from build123d import *

# Parameters (mm, degrees)
BOSS_EXTRUDE1_DEPTH = 20
BOSS_EXTRUDE2_START = 10
BOSS_EXTRUDE2_DEPTH = 10
SKETCH4_R           = 2.6
CUT_EXTRUDE2_DEPTH  = 6
CUT_EXTRUDE3_REACH  = 49.399
SKETCH2_R           = 6.6


with BuildPart() as part:
    # Sketch1 → Boss-Extrude1 (new body)
    with BuildSketch(Plane.XY):
        with BuildLine():
            Line((-33.49686368, 14.646798017), (16.10313632, 14.646798017))
            ThreePointArc((16.10313632, 14.646798017), (16.951664458, 14.295326155), (17.30313632, 13.446798017))
            Line((17.30313632, 13.446798017), (17.30313632, -25.353201983))
            Line((17.30313632, -25.353201983), (-34.69686368, -25.353201983))
            Line((-34.69686368, -25.353201983), (-34.69686368, 13.446798017))
            ThreePointArc((-34.69686368, 13.446798017), (-34.345391817, 14.295326155), (-33.49686368, 14.646798017))
        make_face()
    extrude(amount=-BOSS_EXTRUDE1_DEPTH)

    # Sketch3 → Boss-Extrude2 (add)
    with BuildSketch(Plane.XY.offset(BOSS_EXTRUDE2_START)):
        with BuildLine():
            Line((17.30313632, -25.353201983), (17.30313632, 13.446798017))
            ThreePointArc((17.30313632, 13.446798017), (16.951664458, 14.295326155), (16.10313632, 14.646798017))
            Line((16.10313632, 14.646798017), (-33.49686368, 14.646798017))
            ThreePointArc((-33.49686368, 14.646798017), (-34.345391817, 14.295326155), (-34.69686368, 13.446798017))
            Line((-34.69686368, 13.446798017), (-34.69686368, -25.353201983))
            Line((-34.69686368, -25.353201983), (17.30313632, -25.353201983))
        make_face()
    extrude(amount=-BOSS_EXTRUDE2_DEPTH)

    # Sketch4 → Cut-Extrude2 (cut)
    with BuildSketch(Plane(origin=(0, 14.646798017, 0), x_dir=(1, 0, 0), z_dir=(0, 1, 0))):
        with Locations(Location((-27.29686368, 5, 0), (0, 0, 270))):
            Circle(SKETCH4_R)
        with Locations(Location((-15.69686368, 5, 0), (0, 0, 270))):
            Circle(SKETCH4_R)
        with Locations(Location((-8.69686368, 12, 0), (0, 0, 270))):
            Circle(SKETCH4_R)
        with Locations(Location((-8.69686368, -2, 0), (0, 0, 270))):
            Circle(SKETCH4_R)
        with Locations(Location((-1.69686368, 5, 0), (0, 0, 270))):
            Circle(SKETCH4_R)
        with Locations(Location((9.90313632, 5, 0), (0, 0, 270))):
            Circle(SKETCH4_R)
    extrude(amount=-CUT_EXTRUDE2_DEPTH, mode=Mode.SUBTRACT)

    # Sketch2 → Cut-Extrude3 (cut, up to next)
    with BuildSketch(Plane.XY, mode=Mode.PRIVATE) as cut_extrude3_sk1:
        with Locations((-8.69686368, -5.353201983)):
            Circle(SKETCH2_R)
    cut_extrude3_tool1 = extrude(cut_extrude3_sk1.sketch, amount=-CUT_EXTRUDE3_REACH, mode=Mode.PRIVATE) & part.part
    add(cut_extrude3_tool1.solids().sort_by_distance((-8.696864, -5.353202, 0))[0], mode=Mode.SUBTRACT)


solid = part.part
Could you check a few things on this model? Use its own coordinates, in mm. A direction names the side the tool comes from. Round coordinates to 2 decimals unless told otherwise and drop trailing zeros. Order: outer loops, then holes, each group sorted by start corner. A loop starts at its lowest first (then second) coordinate and runs counter-clockwise, first axis right, second up.
(1) I'm going to push flat-ended pins straight in: pin 1 (12 mm diameter, centred on x = -8.7, y = -5.35, fed in from -Z); pin 2 (4 mm diameter, centred on x = -27.5, z = -4.5, fed in from +Y). Where does each tip first touch, or does it pass through?
Response values:
pin 1: stops at z = 0
pin 2: stops at y = 8.65
(2) Which directions (+Z, -Z, +X, -X, +Y, -Y) give clear straight access to the entire face, cutting with the end or side of a thin tool? Please do faces 1 (the cylindrical face through (-2.6, -7.88, -9.86)), 2 (the cylindrical face through (-0.92, 11.69, -2.52)), 3 (the flat face through (-9, -25.353, -5)).
Response values:
face 1: -Z
face 2: +Y
face 3: +Z, -Z, +X, -X, -Y
(3) Imagine slicing it at B-B (y = 9.5). Write out the boundary of the cut face in (x, z).
Response values:
outline: (-34.7, -20) - (17.3, -20) - (17.3, 10) - (-34.7, 10) - close; hole circle Ø5.2 at (-27.3, -5); hole circle Ø5.2 at (-15.7, -5); hole circle Ø5.2 at (-8.7, -12); hole circle Ø5.2 at (-8.7, 2); hole circle Ø5.2 at (-1.7, -5); hole circle Ø5.2 at (9.9, -5)
(4) Imagine slicing it at D-D (y = -3.5). Write out the boundary of the cut face in (x, z).
Response values:
outline: (-34.7, -20) - (-15.03, -20) - (-15.03, 0) - (-2.36, 0) - (-2.36, -20) - (17.3, -20) - (17.3, 10) - (-34.7, 10) - close
(5) If we mould it in two halves opening along X, with no side actions, what happens to faces 4 (the flat face through (-8, 14.647, -5)), 5 (the flat face through (17.303, -6, -5)), 6 (the cylindrical face through (-10.28, 11.69, -0.06))? For each: released by +X, released by -X, zero draft, split by the parting line, or undercut.
Response values:
face 4: zero draft
face 5: released by +X
face 6: undercut
(6) Imagine slicing it at A-A (z = 2). Write out the boundary of the cut face in (x, y), plus the area to 3 significant figures.
Response values:
outline: (-34.7, -25.35) - (17.3, -25.35) - (17.3, 13.45) arc R1.2 ccw to (16.1, 14.65) - (-6.1, 14.65) - (-6.1, 8.65) - (-11.3, 8.65) - (-11.3, 14.65) - (-33.5, 14.65) arc R1.2 ccw to (-34.7, 13.45) - close
area: 2,050 mm2
(7) Imagine slicing it at C-C (z = -12). Write out the boundary of the cut face in (x, y), plus the area to 3 significant figures.
Response values:
outline: (-34.7, -25.35) - (17.3, -25.35) - (17.3, 13.45) arc R1.2 ccw to (16.1, 14.65) - (-6.1, 14.65) - (-6.1, 8.65) - (-11.3, 8.65) - (-11.3, 14.65) - (-33.5, 14.65) arc R1.2 ccw to (-34.7, 13.45) - close; hole circle Ø13.2 at (-8.7, -5.35)
area: 1,910 mm2
(8) Please list where these lines run through material, in increasing order: line 1 along X through (y, z) = (12.9, -5); line 2 along X through (y, z) = (11.85, -12); line 3 along Y through (x, z) = (-9, -8.5).
Response values:
line 1: x = -34.7 to -29.9, -24.7 to -18.3, -13.1 to -4.3, 0.9 to 7.3, 12.5 to 17.3
line 2: x = -34.7 to -11.3, -6.1 to 17.3
line 3: y = -25.35 to -11.95, 1.24 to 14.65
